Autodesk Inventor part; units mm, degrees
ref_plane "Work Plane2" through (0, 0, -2.54) normal (0, 0, -1) x (-1, 0, 0)
ref_plane "YZ Plane" through (0, 0, 0) normal (1, 0, 0) x (0, 1, 0)
ref_plane "XZ Plane" through (0, 0, 0) normal (0, 1, 0) x (-1, 0, 0)
sketch "Sketch1" plane through (0, 0, 0) normal (0, 0, 1) x (1, 0, 0)
  circle A0 centre (0, 0) radius 23.0505
  dimension "d0" = 46.101
extrude "Extrusion1" add sketch "Sketch1" along normal blind 1.5875
sketch "Sketch4" plane through (0, 0, 0) normal (0, 0, -1) x (-1, 0, 0)
  circle A0 centre (0, 0) radius 13.8303
  circle A1 centre (0, 0) radius 23.0505
  dimension "d14" = 27.6606
extrude "Extrusion2" add sketch "Sketch4" along normal blind 2.54 contours A0
ref_plane "Work Plane2" through (0, 0, -2.54) normal (0, 0, -1) x (-1, 0, 0)
mirror "Mirror1" about plane through (0, 0, -2.54) normal (0, 0, -1) of "Extrusion1", "Extrusion2"
sketch "Sketch5" plane through (0, 0, 1.5875) normal (0, 0, 1) x (1, 0, 0)
  point P0 (0, 0)
  point P1 (0, 0)
hole "Hole1" at (0, 0, 1.5875) direction (0, 0, -1) diameter 15.875 end through all
properties part number "CLB_072_ScissorPulley" material "PC/ABS Plastic"
Here's how the part is built. I have some questions about the finished solid (model axes, mm). A direction names the side the tool comes from. Round coordinates to 2 decimals unless told otherwise and drop trailing zeros. Loops run counter-clockwise (first coordinate to the right, second up) from the corner with the lowest first, then second, coordinate; pieces in that order, holes last. Notation, with made-up numbers: (41, 21) -> (67, 21) arc R26 ccw to (67, 51) -> close; hole circle Ø9 at (23.5, 61). An arc over 180 degrees is marked (long way). Answer as CSV lines item,"result".
1. Which directions (+Z, -Z, +X, -X, +Y, -Y) give clear straight access to the entire face, cutting with the end or side of a thin tool? Please do faces 4 (the face through (-13.192, -4.154, -2.504)), 5 (the face through (10, 0, 1.588)).
Final values:
face 4,"none"
face 5,"+Z, +X, -X, +Y, -Y"
2. If I drill on L1, parallel to Z at x = 10.5, y = -13; L2, parallel to Y at x = 0, z = -4.5; L3, parallel to Y at x = 5, z = -3, over which ranges is the centre line in solid material (lowest first)?
Final values:
L1,"z = -6.67 to -5.08, 0 to 1.59"
L2,"y = -13.83 to -7.94, 7.94 to 13.83"
L3,"y = -12.89 to -6.16, 6.16 to 12.89"
3. For pin 1 (4 mm diameter, centred on x = 8, z = -1, fed in from -Y); pin 2 (1 mm diameter, centred on y = 5, z = -1.5, fed in from -X); pin 3 (3 mm diameter, centred on y = -15.5, z = -4.5, fed in from +X); pin 4 (14 mm diameter, centred on x = -1.5, y = 2.5, fed in from +Z), each with a flat end and sliding along its axis, tell me the tip position at first contact or that it passes through.
Final values:
pin 1,"stops at y = -22.18"
pin 2,"stops at x = -13.08"
pin 3,"stops at x = 18.22"
pin 4,"stops at z = 1.59"
4. If we section it at D-D on y = -11: Please give me the cut outline in (x, z), plus the area to 3 significant figures.
Final values:
outline,"(-20.26, -6.67) -> (20.26, -6.67) -> (20.26, -5.08) -> (8.38, -5.08) -> (8.38, 0) -> (20.26, 0) -> (20.26, 1.59) -> (-20.26, 1.59) -> (-20.26, 0) -> (-8.38, 0) -> (-8.38, -5.08) -> (-20.26, -5.08) -> close"
area,"214 mm^2"
5. If we section it at A-A on y = 0: Please give me the cut outline in (x, z).
Final values:
outline,"(-23.05, -6.67) -> (-7.94, -6.67) -> (-7.94, 1.59) -> (-23.05, 1.59) -> (-23.05, 0) -> (-13.83, 0) -> (-13.83, -5.08) -> (-23.05, -5.08) -> close; (7.94, -6.67) -> (23.05, -6.67) -> (23.05, -5.08) -> (13.83, -5.08) -> (13.83, 0) -> (23.05, 0) -> (23.05, 1.59) -> (7.94, 1.59) -> close"
6. If we section it at C-C on z = -1.25: Please give me the cut outline in (x, y) (1 decimal).
Final values:
outline,"circle Ø27.7 at (0, 0); hole circle Ø15.9 at (0, 0)"
7. Thinking about a two-plate mould opening in Z: for faces 1 (the face through (-5, 22.5, 0.8)), 2 (the face through (-10, 0, -6.668)), 3 (the face through (10, -10, 0)), which applies, released by +Z, released by -Z, zero draft, split by the parting line, or undercut?
Final values:
face 1,"zero draft"
face 2,"released by -Z"
face 3,"undercut"
